Build history of the part. All positions in model axes, mm. Face numbers are marked on the shaded views. A direction names the side the tool comes from. Round coordinates to 2 decimals unless told otherwise and drop trailing zeros. Write each loop counter-clockwise with the first axis right and the second up, starting at its lowest first coordinate (ties: lowest second). Pieces come first, ordered by that corner, then holes. Notation, with made-up numbers: (-25, 29.5) -> (-16, 29.5) arc R22 cw to (-16, 67.5) -> close; hole circle Ø9 at (-7.5, 16.5). An arc over 180 degrees is marked (long way). Return JSON: item names as keys, results as strings.
from build123d import *

# Parameters (mm, degrees)
F0_R     = 15.2162229734
F1_DEPTH = 10
F2_R     = 5.1506751803
F3_DEPTH = 10
F4_R     = 4.99999


# Not quite as in the source:
# - a fillet or chamfer is up to 0.001 mm smaller than in the source, because OpenCascade refuses the exact size


with BuildPart() as f1:
    # F0 (on Front) → F1 (new body)
    with BuildSketch(Plane.XZ):
        Circle(F0_R)
    extrude(amount=F1_DEPTH)

    # F2 (on face) → F3 (join)
    with BuildSketch(Plane.XZ.offset(10)):
        Circle(F2_R)
    extrude(amount=F3_DEPTH)

    # F4 (radius 5 in the source; OpenCascade refuses exactly that, so slightly less here)
    f4_edges = [f1.edges().sort_by_distance(p)[0] for p in [
        (15.216223, -5, 0),
        (-15.216223, 0, 0),
        (-15.216223, -10, 0),
    ]]
    fillet(f4_edges, radius=F4_R)


solid = f1.part
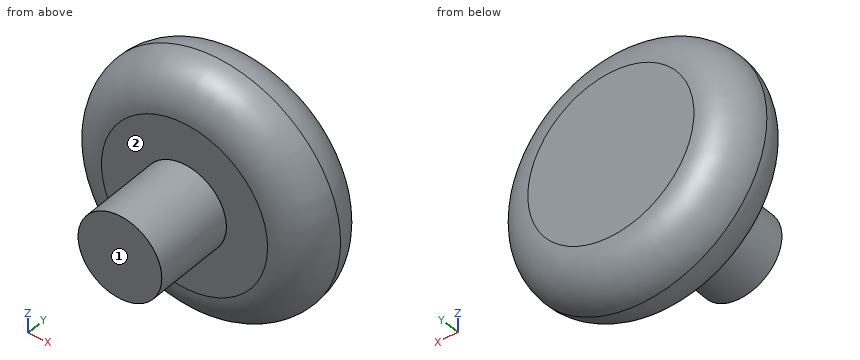
Q1. Saw through at D-D on y = -1.5. List the corners of the cut face in (x, z), then the cut area to 3 significant figures.
Verdict:
{"outline": "circle Ø27.57 at (0, 0)", "area": "597 mm²"}
Q2. Saw through at C-C on y = -14.5. List the corners of the cut face in (x, z), then the cut area to 3 significant figures.
Verdict:
{"outline": "circle Ø10.3 at (0, 0)", "area": "83.3 mm²"}
Q3. Wall check: L1, parallel to Y at x = -8, z = 2; L2, parallel to Z at x = -5, y = -5; L3, parallel to Y at x = -9, z = -10.5. Give the ranges that are in metal, low to high.
Verdict:
{"L1": "y = -10 to 0", "L2": "z = -14.37 to 14.37", "L3": "y = -8.46 to -1.54"}
Q4. Pin check, flat tips, straight feed: pin 1 Ø4 at (x, y) = (1.5, -14.5) entering from -Z; pin 2 Ø1.5 at (y, z) = (-7.5, 1.5) entering from -X; pin 3 Ø12 at (y, z) = (-14.5, 1.5) entering from -X. Stop position of each tip, or through.
Verdict:
{"pin 1": "stops at z = -5.15", "pin 2": "stops at x = -14.83", "pin 3": "stops at x = -13.73"}
Q5. 3-axis set-ups, long thin cutter, end or side, ignore diameter. For the marked faces 1 and 2: which of +Z, -Z, +X, -X, +Y, -Y reach the whole face in a straight line?
Verdict:
{"face 1": "+Z, -Z, +X, -X, -Y", "face 2": "-Y"}
